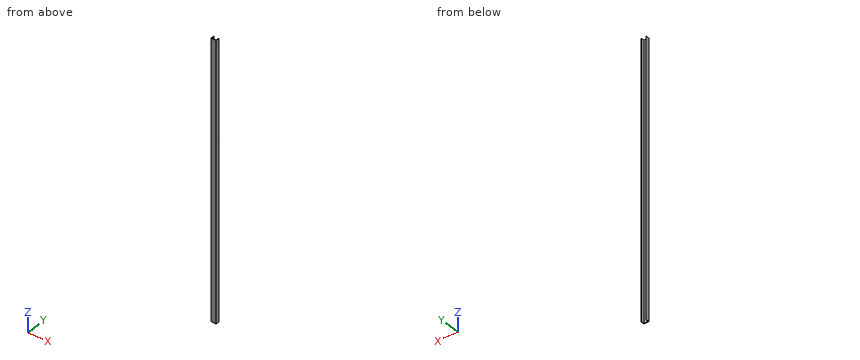
Autodesk Inventor part; units mm, degrees
ref_plane "YZ Plane" through (0, 0, 0) normal (1, 0, 0) x (0, 1, 0)
ref_plane "XZ Plane" through (0, 0, 0) normal (0, 1, 0) x (-1, 0, 0)
ref_plane "XY Plane" through (0, 0, 0) normal (0, 0, 1) x (1, 0, 0)
sketch "Sketch1" plane through (0, 0, 0) normal (0, 0, 1) x (1, 0, 0)
  line L0 (-9.49, 0.83) -> (9.49, 0.83)
  line L1 (11.15, 1.3646) -> (11.15, -0.83)
  line L2 (11.15, -0.83) -> (-11.15, -0.83)
  line L3 (-11.15, -0.83) -> (-11.15, 1.0973)
  line L4 (-9.49, 0.83) -> (-9.49, 13.67)
  line L5 (-9.49, 13.67) -> (-11.15, 13.67)
  line L6 (-11.15, 13.67) -> (-11.15, 1.0973)
  line L7 (9.49, 0.83) -> (9.49, 13.67)
  line L8 (9.49, 13.67) -> (11.15, 13.67)
  line L9 (11.15, 13.67) -> (11.15, 1.3646)
  point P0 (0, 0)
  point P1 (0, 0)
  dimension "d0" = 22.3
  dimension "d1" = 11.15
  dimension "d3" = 0.83
  dimension "d4" = 14.5
  dimension "d5" = 1.66
  dimension "d6" = 1.66
  dimension "d7" = 14.5
  dimension "d10" = 1.66
extrude "Extrusion1" add sketch "Sketch1" along normal mid plane 1220
equation "\"d6\" = d5"
equation "\"d7\" = d4"
equation "\"d10\" = d5"
properties part number "Track"
Geometry check sheet. Reference: the model listing, model coordinates, mm. Round coordinates to 2 decimals unless told otherwise and drop trailing zeros. Write each loop counter-clockwise with the first axis right and the second up, starting at its lowest first coordinate (ties: lowest second). Pieces come first, ordered by that corner, then holes. Notation, with made-up numbers: (61, 13) - (111, 13) arc R23 cw to (111, 22) - close; hole circle Ø5 at (85.5, -18.5). An arc over 180 degrees is marked (long way). Write each question's results on one line, items separated by ' | '.
(1) Thickness scan on probe 1 along X at (y, z) = (12.75, 423.5); probe 2 along Y at (x, z) = (9.25, 8.5). Record the ranges inside material, lowest first. Write a range as from..to.
Computed:
probe 1: x = -11.15..-9.49, 9.49..11.15 | probe 2: y = -0.83..0.83
(2) Sectioned sample at B-B, the plane z = 503.5. Enter the section's corners in (x, y), plus the area to 3 significant figures.
Computed:
outline: (-11.15, -0.83) - (11.15, -0.83) - (11.15, 13.67) - (9.49, 13.67) - (9.49, 0.83) - (-9.49, 0.83) - (-9.49, 13.67) - (-11.15, 13.67) - close | area: 79.6 mm^2
(3) Depth check by flat-ended pin: pin 1 Ø12 at (x, z) = (0.5, 101) entering from +Y. Enter the tip coordinate at first touch or a pass-through.
Computed:
pin 1: stops at y = 0.83
(4) Sectioned sample at C-C, the plane x = -3.25. Enter the section's corners in (y, z), plus the area to 3 significant figures.
Computed:
outline: (-0.83, -610) - (0.83, -610) - (0.83, 610) - (-0.83, 610) - close | area: 2,030 mm^2
(5) Sectioned sample at A-A, the plane y = 9. Enter the section's corners in (x, z).
Computed:
outline: (-11.15, -610) - (-9.49, -610) - (-9.49, 610) - (-11.15, 610) - close; (9.49, -610) - (11.15, -610) - (11.15, 610) - (9.49, 610) - close
